Read the model definition and answer for the solid it produces. Units are mm, in the model's axes. A direction names the side the tool comes from. Round coordinates to 2 decimals unless told otherwise and drop trailing zeros. Write each loop counter-clockwise with the first axis right and the second up, starting at its lowest first coordinate (ties: lowest second). Pieces come first, ordered by that corner, then holes. Notation, with made-up numbers: (67, 16) - (111, 16) arc R28 ccw to (111, 49) - close; hole circle Ø1 at (9, 16). An arc over 180 degrees is marked (long way). Answer as CSV lines item,"result". Start each with the question number.
1) Which of the six approach directions +Z, -Z, +X, -X, +Y, -Y give full straight-line access (tool end or side, diameter ignored) to faces 4 (the flat face through (-1, 44, 0)), 5 (the flat face through (-31, 30, 1))?
2) For a pull along X with two mould halves and no side action, classify faces 1 (the flat face through (-1, 44, 2)), 2 (the flat face through (-30, -31, 1)), 3 (the cylindrical face through (-20.59, 92.74, 0.99)) as +X half, -X half, draft (parallel to the pull), parting line (faces both ways), or undercut.
3) Consider line 1 along Y through (x, z) = (0, 0.75); line 2 along Y through (x, z) = (-1, 1.6); line 3 along X through (y, z) = (-80, 0.85). Determine where each line is inside the solid, lowest interval first.
4) Find section B-B on y = 0. Determine the outline of the cut face in (x, z).
5) Find section D-D on y = -80. Determine the outline of the cut face in (x, z).
6) Each of these flat-tipped pins is pushed along its axis until it touches: pin 1 (1 mm diameter, centred on x = 8, z = 1, fed in from +Y); pin 2 (0.6 mm diameter, centred on x = -9, z = 0.5, fed in from -Y); pin 3 (1 mm diameter, centred on y = -48.5, z = 0.5, fed in from +X). Where does it stop, or does it pass through?
7) Find section A-A on z = 0.45. Determine the outline of the cut face in (x, y), then the cut area to 3 significant figures.
Autodesk Inventor part; units mm, degrees
ref_plane "YZ Plane" through (0, 0, 0) normal (1, 0, 0) x (0, 1, 0)
ref_plane "XZ Plane" through (0, 0, 0) normal (0, 1, 0) x (-1, 0, 0)
ref_plane "XY Plane" through (0, 0, 0) normal (0, 0, 1) x (1, 0, 0)
sketch "Sketch1" plane through (0, 0, 0) normal (0, 0, 1) x (1, 0, 0)
  circle A0 centre (0, 0) radius 95
  line L0 (43, 43) -> (-43, 43)
  line L1 (-43, 43) -> (-43, -43)
  line L2 (-43, -43) -> (43, -43)
  line L3 (43, -43) -> (43, 43)
  line L4 (43, 43) -> (-43, -43) construction
  line L5 (-43, 43) -> (43, -43) construction
  dimension "d157" = 190
  dimension "d158" = 86
  dimension "d159" = 86
extrude "Plate5" add sketch "Sketch1" along normal blind 2
sketch "Sketch7" plane through (0, 0, 0) normal (0, 0, -1) x (-1, 0, 0)
  circle A0 centre (0, 80) radius 8.5
  point P0 (0, 0)
  dimension "d160" = 17
  dimension "d161" = 80
extrude "Cut1" cut sketch "Sketch7" against normal blind 2
pattern_circular "Circular Pattern1" count 4 over 360 about axis through (0, 0, -10) along (0, 0, 1) of "Cut1"
chamfer "Corner Chamfer2" distance 25 angle 45 4 edges at (-43, -43, 1) (43, -43, 1) (-43, 43, 1) (43, 43, 1)
properties part number "PRS 1792 funnel FLANGE 50-90_1000x90_D1200" material "Stainless Steel"
Check values:
1,face 4,"-Z, +X, -X, +Y, -Y"
1,face 5,"+Z, -Z"
2,face 1,"draft"
2,face 2,"undercut"
2,face 3,"parting line"
3,line 1,"y = -95 to -88.5, -71.5 to -43, 43 to 71.5, 88.5 to 95"
3,line 2,"y = -94.99 to -88.44, -71.56 to -43, 43 to 71.56, 88.44 to 94.99"
3,line 3,"x = -51.23 to -8.5, 8.5 to 51.23"
4,outline,"(-95, 0) - (-88.5, 0) - (-88.5, 2) - (-95, 2) - close; (-71.5, 0) - (-43, 0) - (-43, 2) - (-71.5, 2) - close; (43, 0) - (71.5, 0) - (71.5, 2) - (43, 2) - close; (88.5, 0) - (95, 0) - (95, 2) - (88.5, 2) - close"
5,outline,"(-51.23, 0) - (-8.5, 0) - (-8.5, 2) - (-51.23, 2) - close; (8.5, 0) - (51.23, 0) - (51.23, 2) - (8.5, 2) - close"
6,pin 1,"stops at y = 94.7"
6,pin 2,"stops at y = -94.6"
6,pin 3,"stops at x = 81.98"
7,outline,"circle Ø190 at (0, 0); hole circle Ø17 at (-80, 0); hole (-43, -18) - (-18, -43) - (18, -43) - (43, -18) - (43, 18) - (18, 43) - (-18, 43) - (-43, 18) - close; hole circle Ø17 at (0, -80); hole circle Ø17 at (0, 80); hole circle Ø17 at (80, 0)"
7,area,"21,300 mm^2"
